Here's the drawing with two shaded views (mm, measured from the low corner). I have some questions. A direction names the side the tool comes from. Coordinates: 2 decimals unless noted, no trailing zeros. Write each loop counter-clockwise with the first axis right and the second up, starting at its lowest first coordinate (ties: lowest second). Pieces come first, ordered by that corner, then holes. Notation, with made-up numbers: M 5,14.25 L 10,14.25 A14 ccw 10,38.25 Z; hole C -37,-2.5 d9. An arc over 180 degrees is marked long. Use one line per item in the form item = value. Start each with the question number.
1. I want a section at B-B, the plane z = 80. List the corners of the cut face in (x, y) for me.
2. I want a section at A-A, the plane x = 20. List the corners of the cut face in (y, z) for me.
3. I want a section at C-C, the plane z = 42.5. List the corners of the cut face in (x, y) for me.
4. On a 3-axis mill with a long thin cutter (end or side, diameter ignored), from which of +Z, -Z, +X, -X, +Y, -Y can I reach the whole of each face in a straight line? I mean the marked faces 1 and 2. Say none if no direction works.
5. I'm going to push flat-ended pins straight in: pin 1 Ø20 at (x, z) = (20, 50) entering from -Y; pin 2 Ø10 at (x, y) = (34.5, 69) entering from +Z. Where does each tip first touch, or does it pass through?
6. I want a section at D-D, the plane z = 25. List the corners of the cut face in (x, y) for me, plus the area to 3 significant figures.
7. Thinking about a two-plate mould opening in Y: for the marked faces 3, 4 and 5, which applies, released by +Y, released by -Y, zero draft, split by the parting line, or undercut?
8. Please list where these lines run through material, in increasing order: line 1 along Y through (x, z) = (18, 77); line 2 along Z through (x, y) = (8, 6.5); line 3 along Z through (x, y) = (32, 4). Write a range as [from, to].
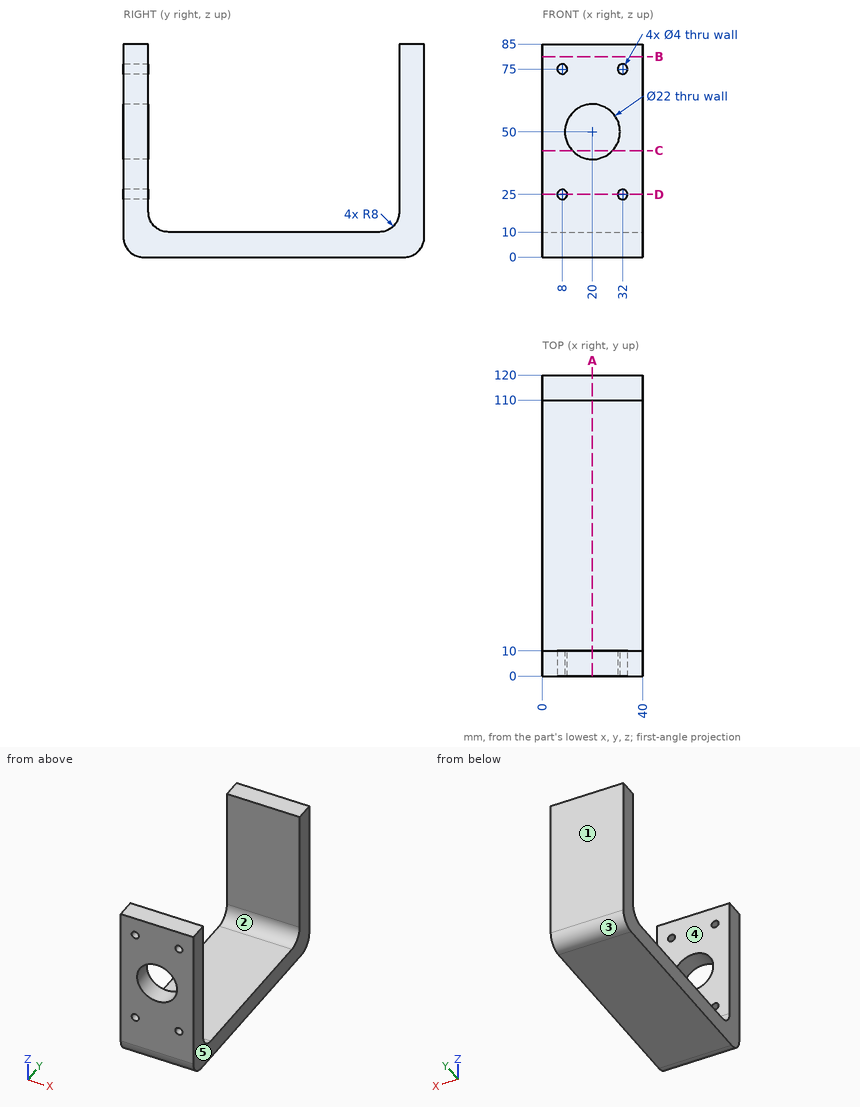
Answer list:
q1.outline = M 0,0 L 40,0 L 40,10 L 0,10 Z; M 0,110 L 40,110 L 40,120 L 0,120 Z
q2.outline = M 0,8 A8 ccw 8,0 L 112,0 A8 ccw 120,8 L 120,85 L 110,85 L 110,18 A8 cw 102,10 L 18,10 A8 cw 10,18 L 10,39 L 0,39 Z; M 0,61 L 10,61 L 10,85 L 0,85 Z
q3.outline = M 0,0 L 11.95,0 L 11.95,10 L 0,10 Z; M 0,110 L 40,110 L 40,120 L 0,120 Z; M 28.05,0 L 40,0 L 40,10 L 28.05,10 Z
q4.face_1 = +Z, -Z, +X, -X, +Y
q4.face_2 = +Z, +X, -X
q5.pin_1 = 110
q5.pin_2 = 10
q6.outline = M 0,0 L 6,0 L 6,10 L 0,10 Z; M 0,110 L 40,110 L 40,120 L 0,120 Z; M 10,0 L 30,0 L 30,10 L 10,10 Z; M 34,0 L 40,0 L 40,10 L 34,10 Z
q6.area = 720 mm²
q7.face_3 = released by +Y
q7.face_4 = undercut
q7.face_5 = zero draft
q8.line_1 = [0, 10], [110, 120]
q8.line_2 = [0.14, 23], [27, 73], [77, 85]
q8.line_3 = [1.07, 23], [27, 73], [77, 85]
